from build123d import *

# Parameters (mm, degrees)
SKETCH1_R           = 4
BOSS_EXTRUDE1_DEPTH = 2
SHELL1_START        = -2
SHELL1_OUTLINE_R    = 4.8
SHELL1_DEPTH        = 3.2


# Read off the part's stored shape, not the designer's step: Shell1
with BuildPart() as part:
    # Sketch1 → Boss-Extrude1 (new, symmetric)
    with BuildSketch(Plane.XY):
        with BuildLine():
            Line((-17.273333042, 5.134508518), (-22.834943086, 4.817083449))
            ThreePointArc((-22.834943086, 4.817083449), (-28.587261134, -1.63159827), (-22.138579415, -7.383916318))
            Line((-22.138579415, -7.383916318), (-16.576969371, -7.066491249))
            ThreePointArc((-16.576969371, -7.066491249), (-0.944763396, -17.995517059), (15.7458991, -8.7634396))
            add(Edge.make_bspline(
                [(15.7458991, -8.7634396), (67.083909385, 4.041585312), (111.853607553, 32.193205755)],
                knots=[0, 0, 0, 1, 1, 1], degree=2))
            ThreePointArc((111.853607553, 32.193205755), (113.10751986, 39.543134952), (105.896265572, 41.438277917))
            add(Edge.make_bspline(
                [(105.896265572, 41.438277917), (63.525953211, 12.424095607), (13.212454281, 12.254071322)],
                knots=[0.987896241, 0.987896241, 0.987896241, 1.987896241, 1.987896241, 1.987896241], degree=2))
            ThreePointArc((13.212454281, 12.254071322), (-4.098137102, 17.548119112), (-17.273333042, 5.134508518))
        make_face()
        with Locations((-22.486761251, -1.283416434)):
            Circle(SKETCH1_R, mode=Mode.SUBTRACT)
        Circle(SKETCH1_R, mode=Mode.SUBTRACT)
        with Locations((108.469927907, 36.408671583)):
            Circle(SKETCH1_R, mode=Mode.SUBTRACT)
    extrude(amount=BOSS_EXTRUDE1_DEPTH, both=True)

    # Shell1 outline → Shell1 (cut)
    with BuildSketch(Plane.XY.offset(SHELL1_START)):
        with BuildLine():
            ThreePointArc((-16.051816298, -6.235216567), (-1.010183418, -17.190644594), (15.211053739, -8.072334002))
            add(Edge.make_bspline(
                [(15.211053739, -8.072334002), (15.222385933, -8.06950746), (15.233718127, -8.066680918), (15.245050322, -8.063854377), (15.256382516, -8.061027835), (15.26771471, -8.058201293), (15.279046904, -8.055374751), (15.290379098, -8.05254821), (15.301711293, -8.049721668), (15.313043487, -8.046895126), (15.324375681, -8.044068584), (15.354121011, -8.036649331), (15.372534147, -8.03205662), (15.390947283, -8.027463909), (15.409360418, -8.022871197), (15.427773554, -8.018278486), (15.44618669, -8.013685775), (15.464599826, -8.009093063), (15.483012962, -8.004500352), (15.501426097, -7.999907641), (15.519839233, -7.995314929), (15.540554011, -7.990148129), (15.542858699, -7.989573289), (15.545136117, -7.989005183), (15.547530208, -7.988408212), (15.549617399, -7.987887312), (15.552237019, -7.987234194), (15.554249413, -7.98673216), (15.556693958, -7.986122386), (15.558944951, -7.985560901), (15.5612476, -7.984986493), (15.56583998, -7.983840868), (15.568136163, -7.983268038), (15.570432338, -7.982695192), (15.572728507, -7.982122328), (15.575024668, -7.981549448), (15.577320821, -7.980976551), (15.579616968, -7.980403637), (15.581913107, -7.979830706), (15.584209239, -7.979257758), (15.586505364, -7.978684793), (15.593393716, -7.976965848), (15.597985921, -7.975819817), (15.602578098, -7.974673718), (15.607170246, -7.973527552), (15.611762364, -7.972381317), (15.616354454, -7.971235016), (15.620946514, -7.970088646), (15.625538546, -7.968942209), (15.630130548, -7.967795704), (15.634722521, -7.966649131), (15.648498354, -7.96320921), (15.657682126, -7.960915659), (15.666865782, -7.958621837), (15.676049322, -7.956327744), (15.685232745, -7.954033381), (15.694416052, -7.951738746), (15.703599244, -7.949443841), (15.712782318, -7.947148666), (15.721965277, -7.944853219), (15.731148119, -7.942557502), (15.77706175, -7.931077562), (15.813790795, -7.921889279), (15.85051798, -7.912696664), (15.887243306, -7.903499717), (15.923966772, -7.894298439), (15.960688378, -7.885092829), (15.997408124, -7.875882887), (16.034126012, -7.866668613), (16.070842039, -7.857450008), (16.107556207, -7.848227071), (16.291117748, -7.802090727), (16.437937227, -7.765112345), (16.584726952, -7.728064656), (16.731486924, -7.690947659), (16.878217144, -7.653761355), (17.02491761, -7.616505744), (17.171588325, -7.579180826), (17.318229287, -7.5417866), (17.464840497, -7.504323068), (17.611421956, -7.466790228), (18.05107708, -7.353983788), (18.34406149, -7.278502266), (18.636926899, -7.202743515), (18.929673307, -7.126707537), (19.222300717, -7.050394331), (19.514809132, -6.973803896), (19.807198553, -6.896936234), (20.099468984, -6.819791344), (20.391620426, -6.742369227), (20.683652882, -6.664669882), (21.559393298, -6.430740165), (22.142744307, -6.273678112), (22.725619399, -6.11550715), (23.308018593, -5.956227279), (23.889941907, -5.795838499), (24.471389362, -5.63434081), (25.052360976, -5.471734213), (25.632856767, -5.308018707), (26.212876755, -5.143194292), (26.792420958, -4.977260969), (28.529626269, -4.476134272), (29.68586008, -4.137614183), (30.84019098, -3.794658457), (31.992619122, -3.447267078), (33.143144661, -3.095440033), (34.29176775, -2.739177308), (35.438488542, -2.378478888), (36.583307191, -2.01334476), (37.726223851, -1.64377491), (38.867238673, -1.269769323), (42.284578093, -0.134445311), (44.55519768, 0.640180196), (46.818211791, 1.432548876), (49.073621643, 2.242661072), (51.32142845, 3.070517125), (53.561633431, 3.916117378), (55.794237801, 4.779462172), (58.019242777, 5.660551849), (60.236649574, 6.559386751), (62.44645941, 7.47596722), (68.878655155, 10.20493448), (73.080612538, 12.065048094), (77.254554243, 13.99063813), (81.400488497, 15.981708647), (85.518423161, 18.038264067), (89.608365726, 20.16030918), (93.67032332, 22.347849143), (97.704302702, 24.600889477), (101.710310261, 26.919436071), (105.688352025, 29.30349518), (109.638433649, 31.753073424)],
                knots=[-0.003323428, -0.003323428, -0.003323428, -0.003323428, -0.003323428, -0.003323428, -0.003323428, -0.003323428, -0.003323428, -0.003323428, -0.003323428, -0.003323428, -0.002109375, -0.002109375, -0.002109375, -0.002109375, -0.002109375, -0.002109375, -0.002109375, -0.002109375, -0.002109375, -0.002109375, -0.000136719, -0.000136719, -0.000136719, -0.000136719, -0.000136719, -0.000136719, -0.000136719, -0.000136719, -0.000136719, -0.000136719, 0.000109863, 0.000109863, 0.000109863, 0.000109863, 0.000109863, 0.000109863, 0.000109863, 0.000109863, 0.000109863, 0.000109863, 0.000356445, 0.000356445, 0.000356445, 0.000356445, 0.000356445, 0.000356445, 0.000356445, 0.000356445, 0.000356445, 0.000356445, 0.000849609, 0.000849609, 0.000849609, 0.000849609, 0.000849609, 0.000849609, 0.000849609, 0.000849609, 0.000849609, 0.000849609, 0.001835937, 0.001835937, 0.001835937, 0.001835937, 0.001835937, 0.001835937, 0.001835937, 0.001835937, 0.001835937, 0.001835937, 0.00578125, 0.00578125, 0.00578125, 0.00578125, 0.00578125, 0.00578125, 0.00578125, 0.00578125, 0.00578125, 0.00578125, 0.0215625, 0.0215625, 0.0215625, 0.0215625, 0.0215625, 0.0215625, 0.0215625, 0.0215625, 0.0215625, 0.0215625, 0.053125, 0.053125, 0.053125, 0.053125, 0.053125, 0.053125, 0.053125, 0.053125, 0.053125, 0.053125, 0.11625, 0.11625, 0.11625, 0.11625, 0.11625, 0.11625, 0.11625, 0.11625, 0.11625, 0.11625, 0.2425, 0.2425, 0.2425, 0.2425, 0.2425, 0.2425, 0.2425, 0.2425, 0.2425, 0.2425, 0.495, 0.495, 0.495, 0.495, 0.495, 0.495, 0.495, 0.495, 0.495, 0.495, 0.979998426, 0.979998426, 0.979998426, 0.979998426, 0.979998426, 0.979998426, 0.979998426, 0.979998426, 0.979998426, 0.979998426, 0.979998426, 0.979998426], degree=11))
            ThreePointArc((109.638433649, 31.753073424), (103.967828672, 38.073334454), (112.386109536, 39.184193417))
            ThreePointArc((112.386109536, 39.184193417), (109.645338699, 41.123948782), (106.30837764, 40.75089845))
            add(Edge.make_bspline(
                [(12.859642213, 11.452874497), (12.875559482, 11.452928286), (12.89147675, 11.452982075), (12.907394019, 11.453035864), (12.923311287, 11.453089654), (12.939228556, 11.453143443), (12.955145825, 11.453197232), (12.971063093, 11.453251021), (12.986980362, 11.45330481), (13.024953461, 11.453433133), (13.047009292, 11.453507666), (13.069065122, 11.453582199), (13.091120953, 11.453656732), (13.113176784, 11.453731266), (13.135232614, 11.453805799), (13.157288445, 11.453880332), (13.179344276, 11.453954865), (13.202778596, 11.454034057), (13.204157085, 11.454038715), (13.205535575, 11.454043373), (13.206914064, 11.454048032), (13.208292554, 11.45405269), (13.209671043, 11.454057348), (13.211049532, 11.454062007), (13.212428022, 11.454066665), (13.215185001, 11.454075982), (13.216554492, 11.454080606), (13.217987164, 11.45408545), (13.219302057, 11.454089949), (13.220750975, 11.45409485), (13.222097481, 11.454099473), (13.223496126, 11.454104254), (13.224878499, 11.454109002), (13.229032762, 11.454123302), (13.231802257, 11.454132885), (13.234571739, 11.454142516), (13.237341208, 11.454152197), (13.240110663, 11.454161926), (13.242880105, 11.454171704), (13.245649534, 11.454181531), (13.248418949, 11.454191408), (13.256727156, 11.454221183), (13.262265907, 11.454241229), (13.267804605, 11.454261471), (13.273343249, 11.454281908), (13.278881841, 11.454302541), (13.284420379, 11.45432337), (13.289958865, 11.454344395), (13.295497296, 11.454365616), (13.312112433, 11.454429865), (13.323188978, 11.45447348), (13.33426531, 11.454517879), (13.345341429, 11.45456306), (13.356417336, 11.454609025), (13.36749303, 11.454655773), (13.378568511, 11.454703304), (13.389643779, 11.454751618), (13.445019058, 11.454997102), (13.489315877, 11.455206018), (13.533609292, 11.455427463), (13.577899303, 11.455661437), (13.62218591, 11.455907939), (13.666469113, 11.45616697), (13.710748913, 11.456438529), (13.755025308, 11.456722618), (13.976390262, 11.458205705), (14.153427758, 11.459592636), (14.330410785, 11.461180031), (14.50733934, 11.46296789), (14.684213418, 11.464956217), (14.861033018, 11.467145013), (15.037798135, 11.469534279), (15.214508768, 11.472124018), (15.7444772, 11.480494658), (16.097571535, 11.486876983), (16.450447892, 11.494061221), (16.803106245, 11.502047384), (17.155546567, 11.510835488), (17.507768833, 11.520425545), (17.859773016, 11.53081757), (18.211559091, 11.542011578), (19.266262913, 11.577999586), (19.968526266, 11.605199584), (20.669916866, 11.635607671), (21.370434487, 11.669223941), (22.070078905, 11.706048488), (22.768849895, 11.746081409), (23.466747231, 11.789322799), (24.163770688, 11.835772751), (26.252218749, 11.984748583), (27.641021145, 12.096900641), (29.026325206, 12.221887985), (30.408128907, 12.359711064), (31.786430221, 12.510370327), (33.161227125, 12.673866223), (34.532517592, 12.850199202), (35.900299598, 13.039369712), (39.993114157, 13.645395185), (42.707615071, 14.100763008), (45.408056156, 14.607483418), (48.094419774, 15.16555678), (50.76668835, 15.774982078), (53.424844378, 16.435756921), (56.068870417, 17.147877537), (58.698749092, 17.911338773), (66.541035798, 20.354212331), (71.711057703, 22.187245864), (76.824392267, 24.225184187), (81.880917363, 26.467954887), (86.880527203, 28.915468978), (91.823134257, 31.567626244), (96.708671175, 34.424320569), (101.53709271, 37.485445273), (106.30837764, 40.75089845)],
                knots=[-0.003533003, -0.003533003, -0.003533003, -0.003533003, -0.003533003, -0.003533003, -0.003533003, -0.003533003, -0.003533003, -0.003533003, -0.002109375, -0.002109375, -0.002109375, -0.002109375, -0.002109375, -0.002109375, -0.002109375, -0.002109375, -0.000136719, -0.000136719, -0.000136719, -0.000136719, -0.000136719, -0.000136719, -0.000136719, -0.000136719, -1.3428e-05, -1.3428e-05, -1.3428e-05, -1.3428e-05, -1.3428e-05, -1.3428e-05, -1.3428e-05, -1.3428e-05, 0.000109863, 0.000109863, 0.000109863, 0.000109863, 0.000109863, 0.000109863, 0.000109863, 0.000109863, 0.000356445, 0.000356445, 0.000356445, 0.000356445, 0.000356445, 0.000356445, 0.000356445, 0.000356445, 0.000849609, 0.000849609, 0.000849609, 0.000849609, 0.000849609, 0.000849609, 0.000849609, 0.000849609, 0.001835937, 0.001835937, 0.001835937, 0.001835937, 0.001835937, 0.001835937, 0.001835937, 0.001835937, 0.00578125, 0.00578125, 0.00578125, 0.00578125, 0.00578125, 0.00578125, 0.00578125, 0.00578125, 0.0215625, 0.0215625, 0.0215625, 0.0215625, 0.0215625, 0.0215625, 0.0215625, 0.0215625, 0.053125, 0.053125, 0.053125, 0.053125, 0.053125, 0.053125, 0.053125, 0.053125, 0.11625, 0.11625, 0.11625, 0.11625, 0.11625, 0.11625, 0.11625, 0.11625, 0.2425, 0.2425, 0.2425, 0.2425, 0.2425, 0.2425, 0.2425, 0.2425, 0.495, 0.495, 0.495, 0.495, 0.495, 0.495, 0.495, 0.495, 0.999531309, 0.999531309, 0.999531309, 0.999531309, 0.999531309, 0.999531309, 0.999531309, 0.999531309, 0.999531309, 0.999531309], degree=9))
            ThreePointArc((12.859642213, 11.452874497), (-4.019017915, 16.744737295), (-16.657009441, 4.368382832))
            Line((-16.657009441, 4.368382832), (-22.789357823, 4.018383265))
            ThreePointArc((-22.789357823, 4.018383265), (-27.78856095, -1.586013006), (-22.184164679, -6.585216134))
            Line((-22.184164679, -6.585216134), (-16.051816298, -6.235216567))
        make_face()
        with Locations((-22.486761251, -1.283416434)):
            Circle(SHELL1_OUTLINE_R, mode=Mode.SUBTRACT)
        Circle(SHELL1_OUTLINE_R, mode=Mode.SUBTRACT)
    extrude(amount=SHELL1_DEPTH, mode=Mode.SUBTRACT)


solid = part.part
Geometry: final body of the model. Coordinates: model frame, mm. A direction names the side the tool comes from. Round coordinates to 2 decimals unless told otherwise and drop trailing zeros. Order: outer loops, then holes, each group sorted by start corner. A loop starts at its lowest first (then second) coordinate and runs counter-clockwise, first axis right, second up.
Q1. Section B-B, the plane y = 0. Give the number of separate pieces and of enclosed holes in the cut face, and give its area (3 significant figures).
Result sheet:
separate pieces: 3
enclosed holes: 0
area: 67.3 mm2
Q2. Section A-A, the plane x = 0. Output: boundary loops of the cut face in (y, z).
Result sheet:
outline: (-18.02, -2) - (-17.22, -2) - (-17.22, 1.2) - (-4.8, 1.2) - (-4.8, -2) - (-4, -2) - (-4, 2) - (-18.02, 2) - close; (4, -2) - (4.8, -2) - (4.8, 1.2) - (17.22, 1.2) - (17.22, -2) - (18.02, -2) - (18.02, 2) - (4, 2) - close
Q3. Material intervals for probe 1 along Y at (x, z) = (0, -0.3); probe 2 along Z at (x, y) = (46.5, 10); probe 3 along X at (y, z) = (6, 0.75), sorted ascending.
Result sheet:
probe 1: y = -18.02 to -17.22, -4.8 to -4, 4 to 4.8, 17.22 to 18.02
probe 2: z = 1.2 to 2
probe 3: x = -16.99 to -16.14, 58.81 to 60.94
Q4. Access query for faces 1 (the face through (-19.397, -7.227, 0.028)), 2 (the face through (-1.285, -17.172, -0.422)), 3 (the face through (-26.483, -1.108, -0.028)). Directions: +Z, -Z, +X, -X, +Y, -Y. A direction counts if a zero-diameter tool reaches every point of the face in a straight line with its end or side. Return the directions, or none.
Result sheet:
face 1: +Z, -Z, -Y
face 2: -Z
face 3: +Z, -Z
